```python
from build123d import *

# Parameters (mm, degrees)
BOSS_EXTRUDE1_DEPTH = 4.9
SKETCH2_R           = 1.45
CUT_EXTRUDE1_DEPTH  = 5.9


with BuildPart() as part:
    # Sketch1 → Boss-Extrude1 (new body)
    with BuildSketch(Plane(origin=(0, 0, 0), x_dir=(0, 0, -1), z_dir=(1, 0, 0))):
        Polygon((0, 0), (0, 4.9), (1.5, 4.9), (1.5, 2.5), (7, 2.5), (7, 0), align=None)
    extrude(amount=BOSS_EXTRUDE1_DEPTH)

    # Sketch2 → Cut-Extrude1 (cut, through all)
    with BuildSketch(Plane.XZ):
        with Locations((2.45, -4.2)):
            Circle(SKETCH2_R)
    extrude(amount=-CUT_EXTRUDE1_DEPTH, mode=Mode.SUBTRACT)


solid = part.part
```
Input: part model. Units: mm. Frame: model coordinates. A direction names the side the tool comes from. Coordinates: 2 decimals unless noted, no trailing zeros. Write each loop counter-clockwise with the first axis right and the second up, starting at its lowest first coordinate (ties: lowest second). Pieces come first, ordered by that corner, then holes. Notation, with made-up numbers: (2, 45) -> (60, 45) arc R25 cw to (60, 65) -> close; hole circle Ø11 at (-14.5, -4.75). An arc over 180 degrees is marked (long way). Write each question's results on one line, items separated by ' | '.
Item 1: Section query A-A on x = 3.5. Return loops of the section in (y, z).
Conclusion:
outline: (0, -7) -> (2.5, -7) -> (2.5, -5.2) -> (0, -5.2) -> close; (0, -3.2) -> (2.5, -3.2) -> (2.5, -1.5) -> (4.9, -1.5) -> (4.9, 0) -> (0, 0) -> close
Item 2: Section query D-D on x = 2.45. Return loops of the section in (y, z), plus the area to 4 significant figures.
Conclusion:
outline: (0, -7) -> (2.5, -7) -> (2.5, -5.65) -> (0, -5.65) -> close; (0, -2.75) -> (2.5, -2.75) -> (2.5, -1.5) -> (4.9, -1.5) -> (4.9, 0) -> (0, 0) -> close | area: 13.85 mm^2
Item 3: Material intervals for probe 1 along Z at (x, y) = (2.45, 0.8); probe 2 along X at (y, z) = (0.4, -4); probe 3 along Y at (x, z) = (3.55, -2), sorted ascending.
Conclusion:
probe 1: z = -7 to -5.65, -2.75 to 0 | probe 2: x = 0 to 1.01, 3.89 to 4.9 | probe 3: y = 0 to 2.5
Item 4: Section query B-B on z = -4.2. Return loops of the section in (x, y).
Conclusion:
outline: (0, 0) -> (1, 0) -> (1, 2.5) -> (0, 2.5) -> close; (3.9, 0) -> (4.9, 0) -> (4.9, 2.5) -> (3.9, 2.5) -> close
Item 5: Section query C-C on y = 0.95. Return loops of the section in (x, z).
Conclusion:
outline: (0, -7) -> (4.9, -7) -> (4.9, 0) -> (0, 0) -> close; hole circle Ø2.9 at (2.45, -4.2)
Item 6: Set-up query: faces 1 (the flat face through (2, 4, -1.5)), 2 (the flat face through (2, 4.9, -1)). Return all of +Z, -Z, +X, -X, +Y, -Y with unobstructed straight access to the full face (end or side cutting, diameter ignored); none if empty.
Conclusion:
face 1: -Z, +X, -X, +Y | face 2: +Z, -Z, +X, -X, +Y
Item 7: Pin query (flat end, axial travel): pin 1 Ø2 at (x, z) = (3.5, -4) entering from +Y; pin 2 Ø2.5 at (x, z) = (2.45, -4.2) entering from -Y; pin 3 Ø2.5 at (x, y) = (2.5, 4) entering from -Z. Return the tip coordinate at first contact, or that it passes through.
Conclusion:
pin 1: stops at y = 2.5 | pin 2: passes through | pin 3: stops at z = -1.5
